Check sheet for the drawn part. Datum: minimum x, y, z corner. Units: mm. A direction names the side the tool comes from. Coordinates: 2 decimals unless noted, no trailing zeros. Order: outer loops, then holes, each group sorted by start corner. A loop starts at its lowest first (then second) coordinate and runs counter-clockwise, first axis right, second up. Notation, with made-up numbers: M -7.75,-16 L 30.25,-16 A16 ccw 30.25,13 Z; hole C 53.25,-28.5 d8. An arc over 180 degrees is marked long. Return JSON: item names as keys, results as strings. Group by question number.
Q1. Mould release check, pull along X, two halves, no side actions. Record for the marked faces 1 and 2: pulls with the +X half, pulls with the -X half, needs draft (parallel to the pull), parting line crosses it, or undercut.
Q2. Go/stop test with flat-tipped pins: pin 1 Ø1.6 at (x, y) = (5.5, 215) entering from +Z; pin 2 Ø9.5 at (x, z) = (53, 12.5) entering from -Y. Record where each tip stops, or that it passes through.
Q3. Thickness scan on probe 1 along Y at (x, z) = (5, 6.5); probe 2 along X at (y, z) = (215, 11); probe 3 along Y at (x, z) = (101.5, 6.5). Record the ranges inside material, lowest first.
Q4. Section check A-A, the plane x = 56. Enter the section's corners in (y, z).
Q5. Access from +Z, -Z, +X, -X, +Y, -Y to the whole of each face (thin tool, end or side, straight path). Record for the marked faces 3 and 4.
Q6. Section check B-B, the plane y = 149. Enter the section's corners in (x, z).
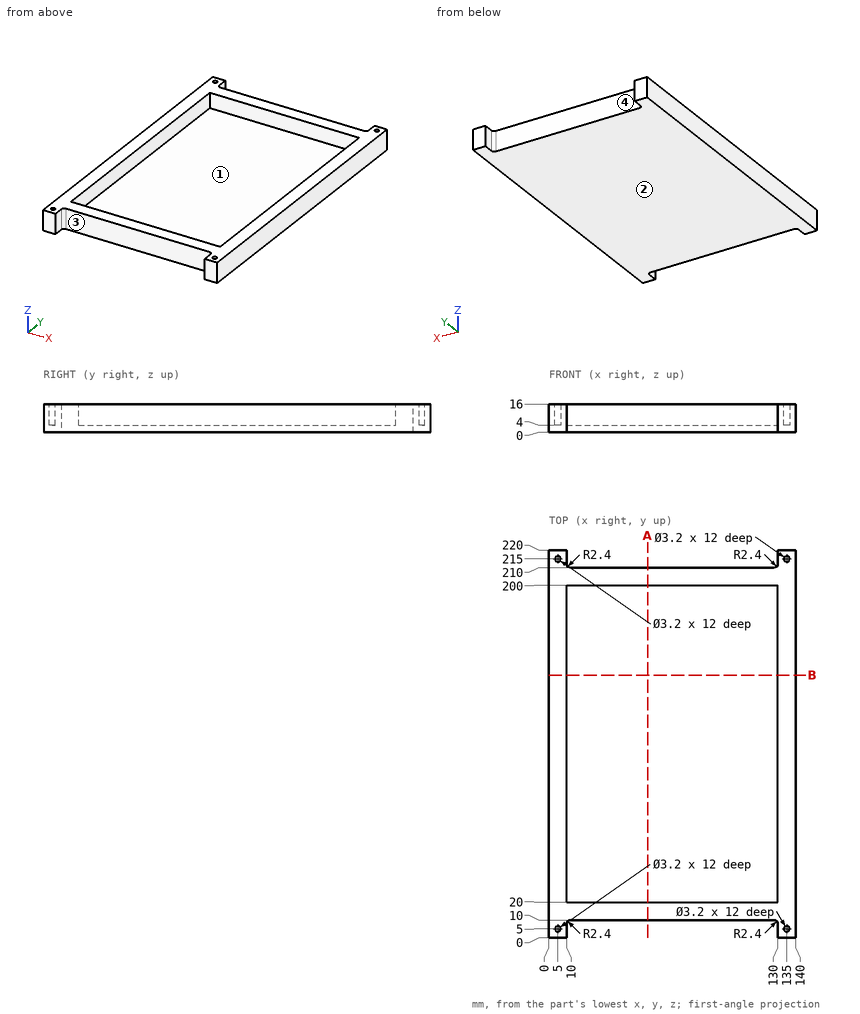
Numbers:
{
 "1": {"face 1": "undercut", "face 2": "needs draft"},
 "2": {"pin 1": "stops at z = 4", "pin 2": "stops at y = 10"},
 "3": {"probe 1": "y = 0 to 3.4, 6.6 to 213.4, 216.6 to 220", "probe 2": "x = 0 to 3.4, 6.6 to 10, 130 to 133.4, 136.6 to 140", "probe 3": "y = 10 to 20, 200 to 210"},
 "4": {"outline": "M 10,0 L 210,0 L 210,16 L 200,16 L 200,4 L 20,4 L 20,16 L 10,16 Z"},
 "5": {"face 3": "+Z, -Z, -Y", "face 4": "+Z, -Z, +Y"},
 "6": {"outline": "M 0,0 L 140,0 L 140,16 L 130,16 L 130,4 L 10,4 L 10,16 L 0,16 Z"}
}
